```python
from build123d import *

# Parameters (mm, degrees)
SKETCH1_W                = 114
SKETCH1_H                = 214
BOSS_EXTRUDE1_DEPTH      = 50
SKETCH4_W                = 25
SKETCH4_H                = 25
CUT_EXTRUDE1_DEPTH       = 248.572211688
SHELL1_START             = 2
SHELL1_OUTLINE_W         = 110
SHELL1_OUTLINE_H         = 185
SHELL1_DEPTH             = 46
SHELL1_2_OUTLINE_W       = 110
SHELL1_2_OUTLINE_H       = 27
SHELL1_2_DEPTH           = 23
M4_CLEARANCE_HOLE1_D     = 4.3
M4_CLEARANCE_HOLE1_DEPTH = 4
M4_CLEARANCE_HOLE1_TIP   = 1.291850331


# Read off the part's stored shape, not the designer's step: Shell1
with BuildPart() as part:
    # Sketch1 → Boss-Extrude1 (new body)
    with BuildSketch(Plane(origin=(0, 0, 0), x_dir=(1, 0, 0), z_dir=(0, 1, 0))):
        with Locations((57, 107)):
            Rectangle(SKETCH1_W, SKETCH1_H)
    extrude(amount=BOSS_EXTRUDE1_DEPTH)

    # Sketch4 → Cut-Extrude1 (cut, through all)
    with BuildSketch(Plane(origin=(114, 0, 0), x_dir=(0, 0, -1), z_dir=(1, 0, 0))):
        with Locations((201.5, 37.5)):
            Rectangle(SKETCH4_W, SKETCH4_H)
    extrude(amount=-CUT_EXTRUDE1_DEPTH, mode=Mode.SUBTRACT)

    # Shell1 outline → Shell1 (cut)
    with BuildSketch(Plane(origin=(0, 0, 0), x_dir=(1, 0, 0), z_dir=(0, 1, 0)).offset(SHELL1_START)):
        with Locations((57, 94.5)):
            Rectangle(SHELL1_OUTLINE_W, SHELL1_OUTLINE_H)
    extrude(amount=SHELL1_DEPTH, mode=Mode.SUBTRACT)

    # Shell1 2 outline → Shell1 2 (cut)
    with BuildSketch(Plane(origin=(0, 0, 0), x_dir=(1, 0, 0), z_dir=(0, 1, 0)).offset(SHELL1_START)):
        with Locations((57, 200.5)):
            Rectangle(SHELL1_2_OUTLINE_W, SHELL1_2_OUTLINE_H)
    extrude(amount=SHELL1_2_DEPTH, mode=Mode.SUBTRACT)

    # M4 Clearance Hole1
    with Locations(Plane(origin=(0, 0, 0), x_dir=(-1, 0, 0), z_dir=(0, -1, 0))):
        with Locations((-32, 32), (-57, 107), (-32, 182), (-82, 32), (-82, 182)):
            Hole(M4_CLEARANCE_HOLE1_D / 2, depth=M4_CLEARANCE_HOLE1_DEPTH)
            with Locations((0, 0, -(M4_CLEARANCE_HOLE1_DEPTH + M4_CLEARANCE_HOLE1_TIP / 2))):  # 118° drill point
                Cone(0, M4_CLEARANCE_HOLE1_D / 2, M4_CLEARANCE_HOLE1_TIP, mode=Mode.SUBTRACT)


solid = part.part
```
Input: part model. Units: mm. Frame: model coordinates. A direction names the side the tool comes from. Coordinates: 2 decimals unless noted, no trailing zeros. Order: outer loops, then holes, each group sorted by start corner. A loop starts at its lowest first (then second) coordinate and runs counter-clockwise, first axis right, second up. Notation, with made-up numbers: (-4, -38.75) - (50, -38.75) arc R19 cw to (50, -18.75) - close; hole circle Ø6 at (49.25, 55). An arc over 180 degrees is marked (long way). Return JSON: item names as keys, results as strings.
Q1. Cut plane C-C (z = -182). Return loops of the section in (x, y).
The answers:
{"outline": "(0, 0) - (29.85, 0) - (29.85, 2) - (2, 2) - (2, 48) - (112, 48) - (112, 2) - (84.15, 2) - (84.15, 0) - (114, 0) - (114, 50) - (0, 50) - close; (34.15, 0) - (79.85, 0) - (79.85, 2) - (34.15, 2) - close"}
Q2. First-contact query: pin 1 (0.6 mm diameter, centred on x = 40, z = -188, fed in from -Y); pin 2 (8 mm diameter, centred on x = 66.5, y = 10.5, fed in from -Z); pin 3 (2 mm diameter, centred on x = 113.5, z = -200, fed in from +Y); pin 4 (4 mm diameter, centred on x = 64, y = 36.5, fed in from -Z). Flat tips, straight axial feed; report the tip coordinate or a pass-through.
The answers:
{"pin 1": "stops at y = 0", "pin 2": "stops at z = -2", "pin 3": "stops at y = 25", "pin 4": "stops at z = -189"}
Q3. Cut plane D-D (y = 37.5). Return loops of the section in (x, z), then the cut area to 3 significant figures.
The answers:
{"outline": "(0, -189) - (114, -189) - (114, 0) - (0, 0) - close; hole (2, -187) - (112, -187) - (112, -2) - (2, -2) - close", "area": "1,200 mm2"}
Q4. Ray query, probe 1 along Z at (x, y) = (32, 1.45); probe 2 along X at (y, z) = (0.9, -32); probe 3 along X at (y, z) = (20.5, -103). Return the intervals inside material, ascending.
The answers:
{"probe 1": "z = -214 to -184.15, -179.85 to -34.15, -29.85 to 0", "probe 2": "x = 0 to 29.85, 34.15 to 79.85, 84.15 to 114", "probe 3": "x = 0 to 2, 112 to 114"}
Q5. Cut plane A-A (z = -98). Return loops of the section in (x, y), then the cut area to 3 significant figures.
The answers:
{"outline": "(0, 0) - (114, 0) - (114, 50) - (0, 50) - close; hole (2, 2) - (112, 2) - (112, 48) - (2, 48) - close", "area": "640 mm2"}
Q6. Access query for faces 4 (the cylindrical face through (56.53, 1.01, -104.9)), 5 (the flat face through (56, 48, -96)), 6 (the flat face through (58, 37, -189)). Directions: +Z, -Z, +X, -X, +Y, -Y. A direction counts if a zero-diameter tool reaches every point of the face in a straight line with its end or side. Return the directions, or none.
The answers:
{"face 4": "-Y", "face 5": "none", "face 6": "-Z, +X, -X, +Y"}
Q7. Draft query along Y for faces 1 (the cylindrical face through (31.53, 1.01, -179.9)), 2 (the flat face through (56, 50, -96)), 3 (the flat face through (56, 25, -2)). Return one class per face: +Y half, -Y half, draft (parallel to the pull), parting line (faces both ways), or undercut.
The answers:
{"face 1": "draft", "face 2": "+Y half", "face 3": "undercut"}
Q8. Cut plane B-B (x = 82). Return loops of the section in (y, z), then the cut area to 3 significant figures.
The answers:
{"outline": "(0, -214) - (2, -214) - (2, -184.15) - (0, -184.15) - close; (0, -179.85) - (2, -179.85) - (2, -34.15) - (0, -34.15) - close; (0, -29.85) - (2, -29.85) - (2, -2) - (48, -2) - (48, -187) - (25, -187) - (25, -189) - (50, -189) - (50, 0) - (0, 0) - close", "area": "927 mm2"}
